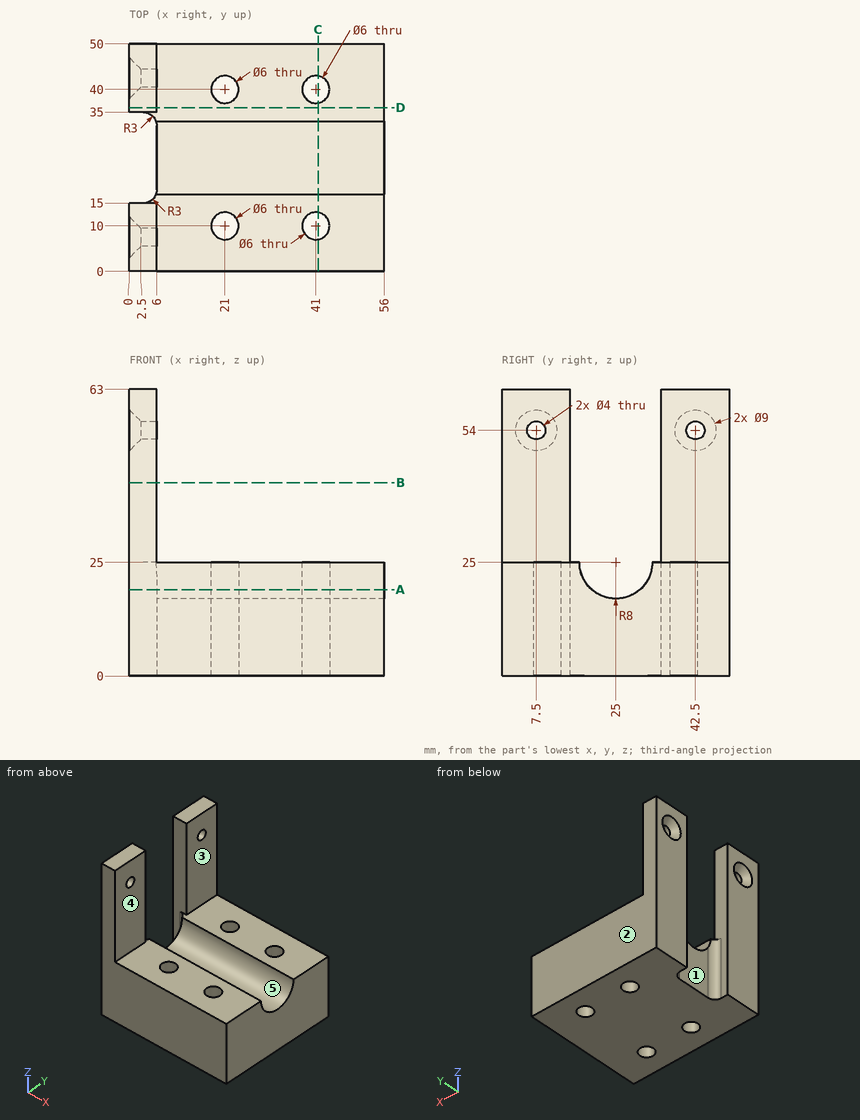
Source: three-view drawing plus pictorial views. Frame: mm from the lowest corner of the part. A direction names the side the tool comes from. Give positions to 0.01 mm unless a question says otherwise; leave off trailing zeros. Loops run counter-clockwise (first coordinate to the right, second up) from the corner with the lowest first, then second, coordinate; pieces in that order, holes last. Notation, with made-up numbers: M 68.25,48 L 111.25,48 A27 cw 111.25,77 Z; hole C 21,56 d5. An arc over 180 degrees is marked long. Put each result on its own line as item: value.
Q1. Pin query (flat end, axial travel): P1, Ø7.5, axis at y = 43.5, z = 52, coming from the +X side; P2, Ø5, axis at y = 42.5, z = 54, coming from the -X side; P3, Ø13.5, axis at x = 39, y = 37.5, coming from the +Z side. Return the tip coordinate at first contact, or that it passes through.
Response values:
P1: stops at x = 6
P2: stops at x = 2
P3: stops at z = 25
Q2. Section C-C (x = 41.5). Return the cut outline in (y, z), and give its area (3 significant figures).
Response values:
outline: M 0,0 L 7.04,0 L 7.04,25 L 0,25 Z; M 12.96,0 L 37.04,0 L 37.04,25 L 33,25 A8 cw 17,25 L 12.96,25 Z; M 42.96,0 L 50,0 L 50,25 L 42.96,25 Z
area: 854 mm²
Q3. Section B-B (z = 42.5). Return the cut outline in (x, y), and give its area (3 significant figures).
Response values:
outline: M 0,0 L 6,0 L 6,15 L 0,15 Z; M 0,35 L 6,35 L 6,50 L 0,50 Z
area: 180 mm²
Q4. Mould query, pull axis Y, two halves, no side actions, for the marked faces 1, 2 and 3. Classes: released by +Y, released by -Y, zero draft, split by the parting line, or undercut.
Response values:
face 1: undercut
face 2: released by +Y
face 3: zero draft
Q5. Section D-D (y = 36). Return the cut outline in (x, z).
Response values:
outline: M 0,0 L 56,0 L 56,25 L 6,25 L 6,63 L 0,63 Z
Q6. Reachability of the marked faces 4 and 5 from +Z, -Z, +X, -X, +Y, -Y: full face, straight path, thin tool, end or side. Return the list, or none.
Response values:
face 4: +Z, +X, +Y, -Y
face 5: +Z, +X, -X
Q7. Line query: probe 1 along Y at (x, z) = (4.6, 54); probe 2 along Y at (x, z) = (21, 8.5); probe 3 along X at (y, z) = (5, 45.5). Output: solid intervals per line, ascending. Write a range as [from, to].
Response values:
probe 1: y = [0, 5.5], [9.5, 15], [35, 40.5], [44.5, 50]
probe 2: y = [0, 7], [13, 37], [43, 50]
probe 3: x = [0, 6]
Q8. Section A-A (z = 19). Return the cut outline in (x, y).
Response values:
outline: M 0,0 L 56,0 L 56,19.71 L 6,19.71 L 6,18 A3 cw 3,15 L 0,15 Z; M 0,35 L 3,35 A3 cw 6,32 L 6,30.29 L 56,30.29 L 56,50 L 0,50 Z; hole C 21,10 d6; hole C 21,40 d6; hole C 41,10 d6; hole C 41,40 d6
